Geometry check sheet. Reference: the model listing, model coordinates, mm. Face numbers are marked on the shaded views. A direction names the side the tool comes from. Give positions to 0.01 mm unless a question says otherwise; leave off trailing zeros. Order: outer loops, then holes, each group sorted by start corner. A loop starts at its lowest first (then second) coordinate and runs counter-clockwise, first axis right, second up.
```python
from build123d import *

# Parameters (mm, degrees)
F0_W     = 54
F0_H     = 40
F1_DEPTH = 20
F2_T     = -2
F3_W     = 5
F3_H     = 5
F4_DEPTH = 2


with BuildPart() as f1:
    # F0 (on Top) → F1 (new body)
    with BuildSketch(Plane.XY):
        Rectangle(F0_W, F0_H)
    extrude(amount=F1_DEPTH)

    # F2
    f2_openings = [f1.faces().sort_by_distance(p)[0] for p in [
        (0, 0, 20),
    ]]
    offset(amount=F2_T, openings=f2_openings)

    # F3 (on face) → F4 (cut)
    with BuildSketch(Plane.XZ.offset(20)):
        with Locations((-22, 15)):
            Rectangle(F3_W, F3_H)
        with Locations((-22, 5)):
            Rectangle(F3_W, F3_H)
    extrude(amount=-F4_DEPTH, mode=Mode.SUBTRACT)


solid = f1.part
```
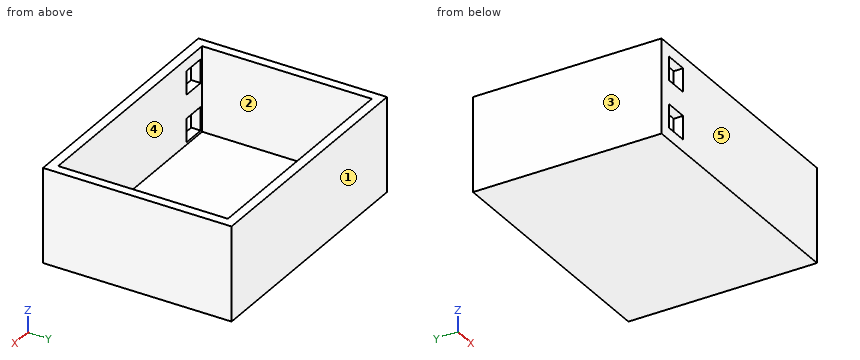
Q1. Cross-section at C-C, the plane y = -14. Record the boundary of the cut face in (x, z), and give its area (3 significant figures).
Q2. Access from +Z, -Z, +X, -X, +Y, -Y to the whole of each face (thin tool, end or side, straight path). Record for the marked faces 4 and 5.
Q3. Cross-section at A-A, the plane x = -21. Record the boundary of the cut face in (y, z), and give its area (3 significant figures).
Q4. Cross-section at B-B, the plane z = 11. Record the boundary of the cut face in (x, y).
Q5. Release check for a two-part mould opening along X. For the marked faces 1, 2 and 3 record: pulls with the +X half, pulls with the -X half, needs draft (parallel to the pull), parting line crosses it, or undercut.
Q6. Thickness scan on L1, parallel to X at y = -17, z = 12.25; L2, parallel to Y at x = -3.5, z = 9; L3, parallel to Z at x = 4.5, y = 12. Record the ranges inside material, lowest first.
Q7. Cross-section at D-D, the plane x = 15. Record the boundary of the cut face in (y, z).
Q8. Gauge pin test, flat end, axial feed: P1, Ø8, axis at x = -17.5, y = 10, coming from the +Z side. Record the tip position at first contact, or that the pin passes through.
Answers follow:
1. outline: (-27, 0) - (27, 0) - (27, 20) - (25, 20) - (25, 2) - (-25, 2) - (-25, 20) - (-27, 20) - close
1. area: 180 mm2
2. face 4: +Z
2. face 5: +Z, -Z, +X, -X, -Y
3. outline: (-20, 0) - (20, 0) - (20, 20) - (18, 20) - (18, 2) - (-18, 2) - (-18, 2.5) - (-20, 2.5) - close; (-20, 7.5) - (-18, 7.5) - (-18, 12.5) - (-20, 12.5) - close; (-20, 17.5) - (-18, 17.5) - (-18, 20) - (-20, 20) - close
3. area: 132 mm2
4. outline: (-27, -20) - (27, -20) - (27, 20) - (-27, 20) - close; hole (-25, -18) - (25, -18) - (25, 18) - (-25, 18) - close
5. face 1: needs draft
5. face 2: undercut
5. face 3: pulls with the -X half
6. L1: x = -27 to -25, 25 to 27
6. L2: y = -20 to -18, 18 to 20
6. L3: z = 0 to 2
7. outline: (-20, 0) - (20, 0) - (20, 20) - (18, 20) - (18, 2) - (-18, 2) - (-18, 20) - (-20, 20) - close
8. P1: stops at z = 2
